Geometry check sheet. Reference: the model listing, model coordinates, mm. A direction names the side the tool comes from. Coordinates: 2 decimals unless noted, no trailing zeros. Order: outer loops, then holes, each group sorted by start corner. A loop starts at its lowest first (then second) coordinate and runs counter-clockwise, first axis right, second up. Notation, with made-up numbers: M 85,10.25 L 114,10.25 A28 ccw 114,44.25 Z; hole C 86,-38 d6. An arc over 180 degrees is marked long. One line per item, written item: value. Start each with the question number.
1) Access from +Z, -Z, +X, -X, +Y, -Y to the whole of each face (thin tool, end or side, straight path). Record for faces 4 (the cylindrical face through (-1.73, -7.81, -5.92)), 5 (the flat face through (-2, 7, 0)).
2) Go/stop test with flat-tipped pins: P1, Ø6, axis at x = -0.5, z = 18.5, coming from the -Y side (3 decimals); P2, Ø1, axis at x = 3.5, z = 14, coming from the +Y side; P3, Ø1, axis at x = 3, z = 30.5, coming from the +Y side. Record where each tip stops, or that it passes through.
3) Draft check along X on faces 1 (the flat face through (2.5, -2.5, 40)), 2 (the cylindrical face through (2.48, -0.78, 13.65)), 3 (the cylindrical face through (5.976, 1.882, 25.003)). Enter one of: pulls with the +X half, pulls with the -X half, needs draft (parallel to the pull), parting line crosses it, or undercut.
4) Sectioned sample at A-A, the plane z = 30. Enter the section's corners in (x, y) (3 decimals).
5) Thickness scan on L1, parallel to X at y = 0, z = 6.5 (3 decimals); L2, parallel to X at y = 0, z = 16 (3 decimals). Record the ranges inside material, lowest first. Write a range as from..to.
```python
from build123d import *

# Parameters (mm, degrees)
F0_R        = 6.665
F0_R_2      = 6.265
F1_DEPTH    = 11
F2_DEPTH    = 40
F0_R_3      = 8
F3_DEPTH    = 12
F4_R        = 2.6
F5_DEPTH    = 52
F6_S5_R     = 6.265
F6_T6_DEPTH = 11
F7_R        = 0.5
F8_R        = 0.5


# Not quite as in the source:
# - a fillet or chamfer that OpenCascade refuses, or shapes differently, is made with other operations: its cross-section is extruded or revolved along the edge and cut away or added


with BuildPart() as f1:
    # F0 (on Top) → F1 (new body)
    with BuildSketch(Plane.XY):
        Circle(F0_R)
        Circle(F0_R_2, mode=Mode.SUBTRACT)
        Circle(F0_R_2)
    extrude(amount=F1_DEPTH)

    # F0 (on Top) → F2 (join)
    with BuildSketch(Plane.XY):
        Circle(F0_R_2)
    extrude(amount=F2_DEPTH)

    # F0 (on Top) → F3 (join)
    with BuildSketch(Plane.XY):
        Circle(F0_R_3)
        Circle(F0_R, mode=Mode.SUBTRACT)
        Circle(F0_R)
        Circle(F0_R_2, mode=Mode.SUBTRACT)
        Circle(F0_R_2)
    extrude(amount=-F3_DEPTH)

    # F4 (on face) → F5 (cut)
    with BuildSketch(Plane(origin=(0, 0, -12), x_dir=(1, 0, 0), z_dir=(0, 0, -1))):
        Circle(F4_R)
    extrude(amount=-F5_DEPTH, mode=Mode.SUBTRACT)

    # F6: chamfer of 0.5 on 4 edges, made by hand


with BuildPart() as f6_tool2:
    # F6_s3 → F6_t4 (revolve)
    with BuildSketch(Plane.XZ):
        Polygon((6.665, 10.5), (6.165, 11), (6.665, 11), align=None)
    revolve(axis=Axis((0, 0, 11), (0, 0, 1)))

    # F6_s5 → F6_t6 (cut, symmetric)
    with BuildSketch(Plane.XY.offset(10.8)):
        Circle(F6_S5_R)
    extrude(amount=F6_T6_DEPTH, both=True, mode=Mode.SUBTRACT)


with BuildPart() as f1_1:
    add(f1.part)

    # F6_t1: cut F6_tool2
    add(f6_tool2.part, mode=Mode.SUBTRACT)

    # F6_s7 → F6_t8 (revolve, cut)
    with BuildSketch(Plane.XZ):
        Polygon((5.765, 40), (6.265, 39.5), (6.265, 40), align=None)
    revolve(axis=Axis((0, 0, 40), (0, 0, 1)), mode=Mode.SUBTRACT)

    # F6_s9 → F6_t10 (revolve, cut)
    with BuildSketch(Plane.XZ):
        Polygon((2.6, 39.5), (3.1, 40), (2.6, 40), align=None)
    revolve(axis=Axis((0, 0, 40), (0, 0, -1)), mode=Mode.SUBTRACT)

    # F6_s11 → F6_t12 (revolve, cut)
    with BuildSketch(Plane.XZ):
        Polygon((3.1, -12), (2.6, -11.5), (2.6, -12), align=None)
    revolve(axis=Axis((0, 0, -12), (0, 0, -1)), mode=Mode.SUBTRACT)

    # F7
    f7_edges = [f1_1.edges().sort_by_distance(p)[0] for p in [
        (-6.665, 0, 10.5),
        (-6.265, 0, 39.5),
        (-2.6, 0, 39.5),
        (-2.6, 0, -11.5),
    ]]
    fillet(f7_edges, radius=F7_R)

    # F8
    f8_edges = [f1_1.edges().sort_by_distance(p)[0] for p in [
        (-6.265, 0, 10.9),
    ]]
    fillet(f8_edges, radius=F8_R)


solid = f1_1.part
```
Final values:
1. face 4: +Z, -Z
1. face 5: +Z
2. P1: stops at y = -6.265
2. P2: stops at y = 5.5
2. P3: stops at y = 5.74
3. face 1: needs draft
3. face 2: undercut
3. face 3: parting line crosses it
4. outline: C 0,0 d12.53; hole C 0,0 d5.2
5. L1: x = -6.665..-2.6, 2.6..6.665
5. L2: x = -6.265..-2.6, 2.6..6.265
